Part model, mm, in its own coordinate system. A direction names the side the tool comes from. Coordinates: 2 decimals unless noted, no trailing zeros. Loops run counter-clockwise (first coordinate to the right, second up) from the corner with the lowest first, then second, coordinate; pieces in that order, holes last. Notation, with made-up numbers: M 29,-31 L 38,-31 A8 cw 38,-18 Z; hole C 59,14 d4. An arc over 180 degrees is marked long. Use a Markdown table: item, result. Add a question column.
1) Pull direction X, two halves, no side cores. Call faces 1 (the flat face through (25.4, -25, 118)), 2 (the flat face through (0, -25, 64)), 3 (the flat face through (89, -25, 127)): released by +X, released by -X, zero draft, split by the parting line, or undercut.
2) Band-saw the part on A-A (z = 44.5). List the corners of the cut face in (x, y).
3) Band-saw the part on D-D (x = 46). List the corners of the cut face in (y, z), plus the area to 3 significant figures.
4) Tool access for faces 4 (the flat face through (50, -25, 0)), 5 (the flat face through (70, -25, 109.602)): list every direction of +Z, -Z, +X, -X, +Y, -Y with a clear straight run to the whole face (end or side of a thin tool).
5) Band-saw the part on C-C (x = 74). List the corners of the cut face in (y, z), plus the area to 3 significant figures.
6) Wall check: probe 1 along X at (y, z) = (-9.5, 117); probe 2 along X at (y, z) = (-22, 101.5); probe 3 along Z at (x, y) = (42, -23). Give the ranges that are in metal, low to high. Write a range as from..to.
7) Pin check, flat tips, straight feed: pin 1 Ø20 at (x, y) = (54, -36) entering from +Z; pin 2 Ø6 at (x, y) = (51.5, -20.5) entering from +Z; pin 3 Ø10 at (x, z) = (47, 40.5) entering from -Y. Stop position of each tip, or through.
8) Band-saw the part on B-B (y = -15.5). List the corners of the cut face in (x, z), plus the area to 3 significant figures.
from build123d import *

# Parameters (mm, degrees)
F1_DEPTH = 50.8
F3_DEPTH = 508


with BuildPart() as f1:
    # F0 (on Front) → F1 (new body)
    with BuildSketch(Plane.XZ):
        Polygon((0, 127), (0, 0), (101.6, 0), (101.6, 127), (76.2, 127), (76.2, 109.6020500779), (63.1024986506, 109.6020500779), (63.1024986506, 90.5520500779), (63.1024986506, 26.5513639897), (38.0738861859, 26.5513639897), (38.0738861859, 90.5520500779), (38.0738861859, 109.6020500779), (25.4, 109.6020500779), (25.4, 127), align=None)
    extrude(amount=F1_DEPTH)

    # F2 (on face) → F3 (cut)
    with BuildSketch(Plane.XY.offset(26.5513639897)):
        with BuildLine():
            Line((63.1024986506, -39.3377331106), (63.1024986506, -9.0668934377))
            ThreePointArc((63.1024986506, -9.0668934377), (50.5881924182, -4.5633521483), (38.0738861859, -9.0668934377))
            Line((38.0738861859, -9.0668934377), (38.0738861859, -39.3377331106))
            ThreePointArc((38.0738861859, -39.3377331106), (50.5881924182, -43.8412744), (63.1024986506, -39.3377331106))
        make_face()
    extrude(amount=F3_DEPTH, mode=Mode.SUBTRACT)


solid = f1.part
Entries:
| question | item | result |
|---|---|---|
| 1 | face 1 | undercut |
| 1 | face 2 | released by -X |
| 1 | face 3 | zero draft |
| 2 | outline | M 0,-50.8 L 38.07,-50.8 L 38.07,0 L 0,0 Z; M 63.1,-50.8 L 101.6,-50.8 L 101.6,0 L 63.1,0 Z |
| 3 | outline | M -50.8,0 L 0,0 L 0,26.55 L -50.8,26.55 Z |
| 3 | area | 1,350 mm2 |
| 4 | face 4 | -Z, +X, -X, +Y, -Y |
| 4 | face 5 | +Z, +Y, -Y |
| 5 | outline | M -50.8,0 L 0,0 L 0,109.6 L -50.8,109.6 Z |
| 5 | area | 5,570 mm2 |
| 6 | probe 1 | 0..25.4, 76.2..101.6 |
| 6 | probe 2 | 0..38.07, 63.1..101.6 |
| 6 | probe 3 | 0..26.55 |
| 7 | pin 1 | z = 109.6 |
| 7 | pin 2 | z = 26.55 |
| 7 | pin 3 | through |
| 8 | outline | M 0,0 L 101.6,0 L 101.6,127 L 76.2,127 L 76.2,109.6 L 63.1,109.6 L 63.1,26.55 L 38.07,26.55 L 38.07,109.6 L 25.4,109.6 L 25.4,127 L 0,127 Z |
| 8 | area | 9,940 mm2 |
